from build123d import *

# Parameters (mm, degrees)
F0_W     = 126.286372
F0_H     = 115.97728
F0_R     = 35.861257
F1_DEPTH = 100
F2_R     = 42.116392
F2_R_2   = 35.861257
F3_DEPTH = 40
F4_R     = 42.482799
F4_R_2   = 35.861257
F5_DEPTH = 40


with BuildPart() as f1:
    # F0 (on Front) → F1 (new body)
    with BuildSketch(Plane.XZ):
        with Locations((0.286363, 0)):
            Rectangle(F0_W, F0_H)
        Circle(F0_R, mode=Mode.SUBTRACT)
    extrude(amount=F1_DEPTH)

    # F2 (on face) → F3 (join)
    with BuildSketch(Plane.XZ.offset(100)):
        Circle(F2_R)
        Circle(F2_R_2, mode=Mode.SUBTRACT)
    extrude(amount=F3_DEPTH)

    # F4 (on face) → F5 (join)
    with BuildSketch(Plane(origin=(0, 0, 0), x_dir=(-1, 0, 0), z_dir=(0, 1, 0))):
        Circle(F4_R)
        Circle(F4_R_2, mode=Mode.SUBTRACT)
    extrude(amount=F5_DEPTH)


solid = f1.part
Model file for the job. Use its own axes, mm. A direction names the side the tool comes from. Round coordinates to 2 decimals unless told otherwise and drop trailing zeros. Order: outer loops, then holes, each group sorted by start corner. A loop starts at its lowest first (then second) coordinate and runs counter-clockwise, first axis right, second up.
(1) Drill centre lines: line 1 (X direction, y = -96.5, z = 0); line 2 (Z direction, x = 0, y = -48.5); line 3 (Z direction, x = 0, y = 15). Where is each one in solid material? Low to high.
(2) Band-saw the part on B-B (x = 0). List the corners of the cut face in (y, z).
(3) Band-saw the part on D-D (z = -47). List the corners of the cut face in (x, y), then the cut area to 3 significant figures.
(4) Band-saw the part on A-A (z = 0). List the corners of the cut face in (x, y), then the cut area to 3 significant figures.
(5) 3-axis set-ups, long thin cutter, end or side, ignore diameter. For faces 1 (the face through (-43, -100, 1)), 2 (the face through (-1, -49, -57.989)), 3 (the face through (31.312, 19.72, 28.712)): which of +Z, -Z, +X, -X, +Y, -Y reach the whole face in a straight line?
(6) Band-saw the part on C-C (y = -6.5). List the corners of the cut face in (x, z), then the cut area to 3 significant figures.
(7) Pin check, flat tips, straight feed: pin 1 (5 mm diameter, centred on x = 36.5, y = -103.5, fed in from +Z); pin 2 (2 mm diameter, centred on x = -46, z = 32, fed in from +Y); pin 3 (10 mm diameter, centred on x = 12, y = -108, fed in from -Z); pin 4 (12 mm diameter, centred on x = 23.5, z = 7, fed in from -Y). Stop position of each tip, or through.
Verdict:
1. line 1: x = -62.86 to -35.86, 35.86 to 63.43
1. line 2: z = -57.99 to -35.86, 35.86 to 57.99
1. line 3: z = -42.48 to -35.86, 35.86 to 42.48
2. outline: (-140, -42.12) - (-100, -42.12) - (-100, -57.99) - (0, -57.99) - (0, -42.48) - (40, -42.48) - (40, -35.86) - (-140, -35.86) - close; (-140, 35.86) - (40, 35.86) - (40, 42.48) - (0, 42.48) - (0, 57.99) - (-100, 57.99) - (-100, 42.12) - (-140, 42.12) - close
3. outline: (-62.86, -100) - (63.43, -100) - (63.43, 0) - (-62.86, 0) - close
3. area: 12,600 mm2
4. outline: (-62.86, -100) - (-42.12, -100) - (-42.12, -140) - (-35.86, -140) - (-35.86, 40) - (-42.48, 40) - (-42.48, 0) - (-62.86, 0) - close; (35.86, -140) - (42.12, -140) - (42.12, -100) - (63.43, -100) - (63.43, 0) - (42.48, 0) - (42.48, 40) - (35.86, 40) - close
4. area: 6,490 mm2
5. face 1: -Y
5. face 2: -Z, +X, -X, +Y, -Y
5. face 3: +Y
6. outline: (-62.86, -57.99) - (63.43, -57.99) - (63.43, 57.99) - (-62.86, 57.99) - close; hole circle Ø71.72 at (0, 0)
6. area: 10,600 mm2
7. pin 1: stops at z = 24.86
7. pin 2: stops at y = 0
7. pin 3: stops at z = -41.53
7. pin 4: passes through
